Build history of the part. All positions in model axes, mm. Round coordinates to 2 decimals unless told otherwise and drop trailing zeros. Write each loop counter-clockwise with the first axis right and the second up, starting at its lowest first coordinate (ties: lowest second). Pieces come first, ordered by that corner, then holes. Notation, with made-up numbers: (44, 5.25) -> (78, 5.25) arc R18 cw to (78, 14.25) -> close; hole circle Ø4 at (-16.75, -40). An arc over 180 degrees is marked (long way). Answer in a Markdown table with one row per item.
```python
from build123d import *

# Parameters (mm, degrees)
F0_W     = 215.9
F0_H     = 279.4
F1_DEPTH = 9.525
F2_W     = 12.7
F2_H     = 96.3083333333
F3_DEPTH = 9.525
F4_R     = 3.175


with BuildPart() as f1:
    # F0 (on Front) → F1 (new body)
    with BuildSketch(Plane.XZ):
        Rectangle(F0_W, F0_H)
    extrude(amount=F1_DEPTH)

    # F2 (on Front) → F3 (join, through all)
    with BuildSketch(Plane.XZ):
        with Locations((114.3, -91.5458333333)):
            Rectangle(F2_W, F2_H)
    extrude(amount=F3_DEPTH)

    # F4
    f4_edges = [f1.edges().sort_by_distance(p)[0] for p in [
        (107.95, -4.7625, 139.7),
        (107.95, -4.7625, -43.391667),
        (120.65, -4.7625, -43.391667),
        (120.65, -4.7625, -139.7),
    ]]
    fillet(f4_edges, radius=F4_R)


solid = f1.part
```
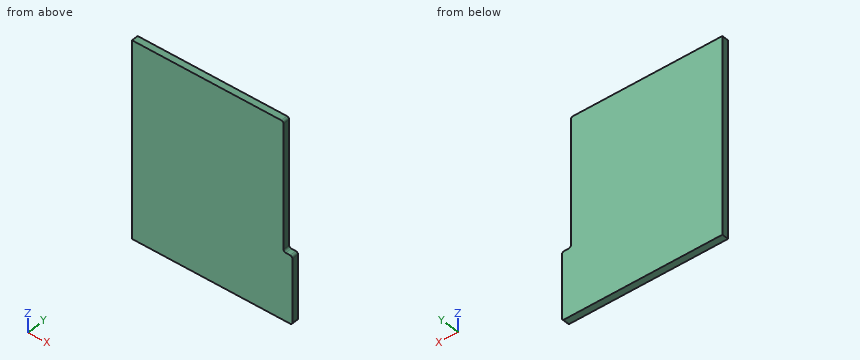
Q1. Wall check: line 1 (X direction, y = -6.75, z = 13.5). Give the ranges that are in metal, low to high. Write a range as [from, to].
A:
| item | result |
|---|---|
| line 1 | [-107.95, 107.95] |
Q2. Drop flat-ended pins along their axis: P1, Ø1.9, axis at x = 115.5, y = -4.5, coming from the +Z side; P2, Ø3, axis at y = -7, z = 7, coming from the +X side. Give the stop position or say it passes through.
A:
| item | result |
|---|---|
| P1 | z = -43.39 |
| P2 | x = 107.95 |
Q3. Saw through at B-B on z = 118. Write the cut outline in (x, y) (3 decimals), plus the area to 3 significant figures.
A:
| item | result |
|---|---|
| outline | (-107.95, -9.525) -> (107.95, -9.525) -> (107.95, 0) -> (-107.95, 0) -> close |
| area | 2,060 mm² |
Q4. Saw through at A-A on y = -4.75. Write the cut outline in (x, z) (3 decimals), plus the area to 3 significant figures.
A:
| item | result |
|---|---|
| outline | (-107.95, -139.7) -> (117.475, -139.7) arc R3.175 ccw to (120.65, -136.525) -> (120.65, -46.567) arc R3.175 ccw to (117.475, -43.392) -> (111.125, -43.392) arc R3.175 cw to (107.95, -40.217) -> (107.95, 136.525) arc R3.175 ccw to (104.775, 139.7) -> (-107.95, 139.7) -> close |
| area | 61,500 mm² |
